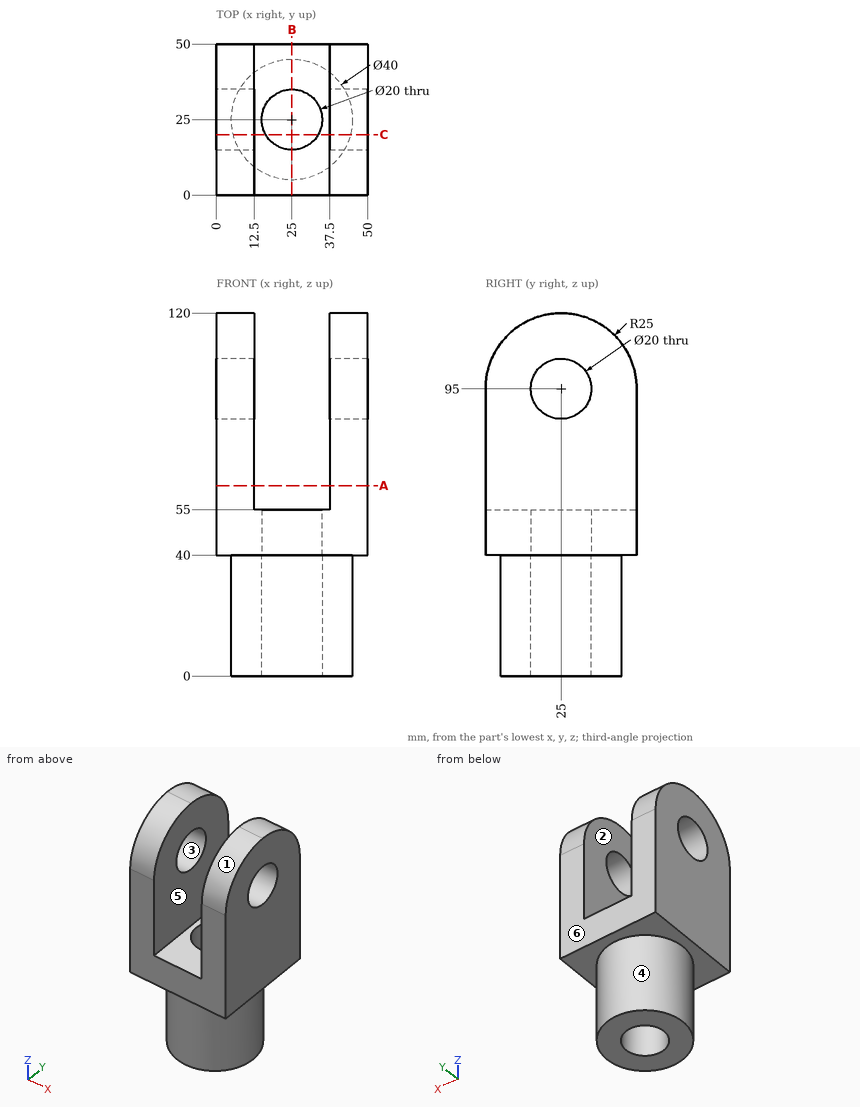
Part print with two shaded views. Sizes in mm from the minimum x, y, z corner. A direction names the side the tool comes from. Round coordinates to 2 decimals unless told otherwise and drop trailing zeros. Order: outer loops, then holes, each group sorted by start corner. A loop starts at its lowest first (then second) coordinate and runs counter-clockwise, first axis right, second up.
(1) 3-axis set-ups, long thin cutter, end or side, ignore diameter. For the marked faces 4, 5 and 6: which of +Z, -Z, +X, -X, +Y, -Y reach the whole face in a straight line?
(2) Pin check, flat tips, straight feed: pin 1 (7.5 mm diameter, centred on x = 26, y = 34, fed in from +Z); pin 2 (2 mm diameter, centred on x = 39.5, y = 17, fed in from +Z); pin 3 (10 mm diameter, centred on x = 28.5, y = 27.5, fed in from -Z); pin 4 (10 mm diameter, centred on x = 11.5, z = 102, fed in from +Y). Stop position of each tip, or through.
(3) Drill centre lines: line 1 (X direction, y = 25, z = 84.5); line 2 (Y direction, x = 25, z = 26); line 3 (Y direction, x = 25, z = 51). Where is each one in solid material? Low to high.
(4) Band-saw the part on A-A (z = 63). List the corners of the cut face in (x, y).
(5) Pull direction Y, two halves, no side cores. Call the marked faces 1, 2 and 3: released by +Y, released by -Y, zero draft, split by the parting line, or undercut.
(6) Band-saw the part on C-C (y = 20). List the corners of the cut face in (x, z).
(7) Band-saw the part on B-B (x = 25). List the corners of the cut face in (y, z).
Verdict:
1. face 4: -Z
1. face 5: +Z, +Y, -Y
1. face 6: +Z, -Z, +X, -X, +Y
2. pin 1: stops at z = 55
2. pin 2: stops at z = 119
2. pin 3: passes through
2. pin 4: stops at y = 49.92
3. line 1: x = 0 to 12.5, 37.5 to 50
3. line 2: y = 5 to 15, 35 to 45
3. line 3: y = 0 to 15, 35 to 50
4. outline: (0, 0) - (12.5, 0) - (12.5, 50) - (0, 50) - close; (37.5, 0) - (50, 0) - (50, 50) - (37.5, 50) - close
5. face 1: released by -Y
5. face 2: zero draft
5. face 3: undercut
6. outline: (0, 40) - (5.64, 40) - (5.64, 0) - (16.34, 0) - (16.34, 55) - (12.5, 55) - (12.5, 86.34) - (0, 86.34) - close; (0, 103.66) - (12.5, 103.66) - (12.5, 119.49) - (0, 119.49) - close; (33.66, 0) - (44.36, 0) - (44.36, 40) - (50, 40) - (50, 86.34) - (37.5, 86.34) - (37.5, 55) - (33.66, 55) - close; (37.5, 103.66) - (50, 103.66) - (50, 119.49) - (37.5, 119.49) - close
7. outline: (0, 40) - (5, 40) - (5, 0) - (15, 0) - (15, 55) - (0, 55) - close; (35, 0) - (45, 0) - (45, 40) - (50, 40) - (50, 55) - (35, 55) - close
